Could you check a few things on this model? Use its own coordinates, in mm. A direction names the side the tool comes from. Coordinates: 2 decimals unless noted, no trailing zeros. Loops run counter-clockwise (first coordinate to the right, second up) from the corner with the lowest first, then second, coordinate; pieces in that order, holes last. Notation, with made-up numbers: (-7.75, 12.25) -> (18.25, 12.25) arc R19 cw to (18.25, 16.25) -> close; hole circle Ø2 at (-23.75, 23). An arc over 180 degrees is marked (long way). One line per question, with ' | ' between items.
from build123d import *

# Parameters (mm, degrees)
SKETCH1_R           = 20
BOSS_EXTRUDE1_DEPTH = 30
SCALE1_SCALE        = 0.1
BOSS_EXTRUDE2_DEPTH = 5.5


with BuildPart() as part:
    # Sketch1 → Boss-Extrude1 (new body)
    with BuildSketch(Plane(origin=(0, 0, 0), x_dir=(1, 0, 0), z_dir=(0, 1, 0))):
        Polygon((17.5, -90), (17.5, 0), (157.5, 0), (157.5, 300), (-157.5, 300), (-157.5, 0), (-72.5, 0), (-72.5, -90), align=None)
        with Locations((-27.5, -55)):
            Circle(SKETCH1_R, mode=Mode.SUBTRACT)
    extrude(amount=BOSS_EXTRUDE1_DEPTH)


with BuildPart() as part_1:
    # Scale1: scaled about (-1.856978843, 15, -136.956329807)
    add(part.part.scale(SCALE1_SCALE).moved(Location((-1.671280959, 13.5, -123.260696826))))

    # Sketch2 → Boss-Extrude2 (add)
    with BuildSketch(Plane.XZ.offset(-13.5)):
        Polygon((-19.421280958, -155.260696826), (-19.421280958, -121.260696826), (-10.921280958, -121.260696826), (-10.921280958, -112.260696826), (2.078719042, -112.260696826), (2.078719042, -121.260696826), (16.078719042, -121.260696826), (16.078719042, -155.260696826), align=None)
        Polygon((14.078719042, -153.260696826), (14.078719042, -123.260696826), (0.078719042, -123.260696826), (0.078719042, -114.260696826), (-8.921280958, -114.260696826), (-8.921280958, -123.260696826), (-17.421280958, -123.260696826), (-17.421280958, -153.260696826), align=None, mode=Mode.SUBTRACT)
    extrude(amount=-BOSS_EXTRUDE2_DEPTH)


solid = part_1.part
1) If we section it at A-A on y = 17.05: Please give me the cut outline in (x, z).
Data:
outline: (-19.42, -155.26) -> (16.08, -155.26) -> (16.08, -121.26) -> (2.08, -121.26) -> (2.08, -112.26) -> (-10.92, -112.26) -> (-10.92, -121.26) -> (-19.42, -121.26) -> close; hole (-17.42, -153.26) -> (14.08, -153.26) -> (14.08, -123.26) -> (0.08, -123.26) -> (0.08, -114.26) -> (-8.92, -114.26) -> (-8.92, -123.26) -> (-17.42, -123.26) -> close
2) I'm going to push flat-ended pins straight in: pin 1 Ø1 at (x, y) = (3.5, 17.5) entering from +Z; pin 2 Ø0.8 at (y, z) = (18.5, -120) entering from +X; pin 3 Ø1.5 at (x, z) = (10.5, -138.5) entering from +Y. Where does each tip first touch, or does it pass through?
Data:
pin 1: z = -121.26 | pin 2: x = 2.08 | pin 3: y = 16.5
3) If we section it at C-C on x = -10: Please give me the cut outline in (y, z), and give its area (4 significant figures).
Data:
outline: (13.5, -155.26) -> (19, -155.26) -> (19, -153.26) -> (16.5, -153.26) -> (16.5, -123.26) -> (19, -123.26) -> (19, -112.26) -> (13.5, -112.26) -> close | area: 161.5 mm²
4) I need wall thicknesses on line 1 along Z through (x, y) = (11.5, 17.9); line 2 along Z through (x, y) = (1, 17.1); line 3 along X through (y, z) = (16.6, -150). Which ranges of each line are inside material? Lowest first, please. Write a range as from..to.
Data:
line 1: -155.26..-153.26, -123.26..-121.26 | line 2: -155.26..-153.26, -123.26..-112.26 | line 3: -19.42..-17.42, 14.08..16.08
5) On a 3-axis mill with a long thin cutter (end or side, diameter ignored), from which of +Z, -Z, +X, -X, +Y, -Y can I reach the whole of each face in a straight line? I mean faces 4 (the face through (16.079, 16, -138)), 5 (the face through (-15, 16, -121.261)), 6 (the face through (14.079, 18, -138)), 7 (the face through (2.079, 16, -117)). Say none if no direction works.
Data:
face 4: +Z, -Z, +X, +Y, -Y | face 5: +Z, -X, +Y, -Y | face 6: +Y | face 7: +Z, +X, +Y, -Y
6) We'd pull the mould along Z, two halves only. Please class faces 1 (the face through (-1, 13.5, -138)), 2 (the face through (-2, 16.5, -138)), 3 (the face through (9, 16, -121.261)): pulls with the +Z half, pulls with the -Z half, needs draft (parallel to the pull), parting line crosses it, or undercut.
Data:
face 1: needs draft | face 2: undercut | face 3: pulls with the +Z half
7) If we section it at B-B on z = -148: Please give me the cut outline in (x, y).
Data:
outline: (-19.42, 13.5) -> (16.08, 13.5) -> (16.08, 19) -> (14.08, 19) -> (14.08, 16.5) -> (-17.42, 16.5) -> (-17.42, 19) -> (-19.42, 19) -> close
